The listing builds one solid part. Answer for the finished solid, in the listing's coordinates (mm). Face numbers are marked on the shaded views. A direction names the side the tool comes from. Give positions to 0.01 mm unless a question says otherwise; leave off trailing zeros. Order: outer loops, then holes, each group sorted by start corner. A loop starts at its lowest first (then second) coordinate and runs counter-clockwise, first axis right, second up. Notation, with made-up numbers: (2.5, 1.5) - (58.5, 1.5) arc R34 ccw to (58.5, 38.5) - close; hole circle Ø9 at (80, 64.5). An arc over 180 degrees is marked (long way). Write each question's results on one line, items separated by ' | '. Start each with the question number.
1. Section A-A (z = 13) is taken. Give the vertices of the cut face in (x, y).
2. Which of the six approach directions +Z, -Z, +X, -X, +Y, -Y give full straight-line access (tool end or side, diameter ignored) to the marked faces 1 and 2?
3. Determine the mould class of the marked faces 3, 4, 5 and 6 for opening direction Y: released by +Y, released by -Y, zero draft, split by the parting line, or undercut.
4. Section C-C (x = -5.5) is taken. Give the vertices of the cut face in (y, z), and give its area (3 significant figures).
5. Section D-D (x = -0.25) is taken. Give the vertices of the cut face in (y, z), and give its area (3 significant figures).
6. A flat-ended cylindrical pin translates along its axis: pin 1 (2 mm diameter, centred on y = -0.5, z = 9.5, fed in from -X). Find the tip coordinate at first contact, or state that the pin passes through.
7. Section B-B (y = 0) is taken. Give the vertices of the cut face in (x, z).
8. Find the intervals of material crossed by L1, parallel to Y at x = 6.6, z = 13; L2, parallel to Z at x = 2.75, y = 0.5, in increasing order.
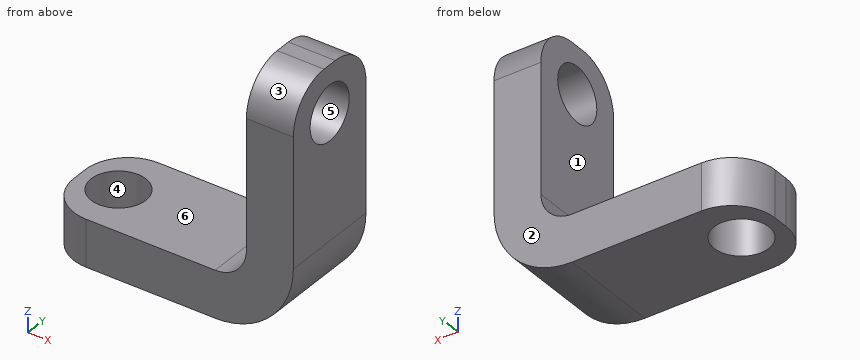
from build123d import *

# Parameters (mm, degrees)
ESQUISSE1_W             = 13
ESQUISSE1_H             = 6.5
ESQUISSE1_R             = 1.75
BOSS_EXTRU_1_DEPTH      = 3
ESQUISSE1_3_W           = 3
ESQUISSE1_3_H           = 6.5
BOSS_EXTRU_2_DEPTH      = 16
ENL_V_MAT_EXTRU_1_REACH = 18
ESQUISSE2_R             = 1.75
CONG_1_R                = 2.75
CONG_2_R                = 2
CONG_3_R                = 5


with BuildPart() as part:
    # Esquisse1 → Boss.-Extru.1 (new body)
    with BuildSketch(Plane.XY):
        with Locations((-1.5, 0)):
            Rectangle(ESQUISSE1_W, ESQUISSE1_H)
        with Locations((-5.5, 0)):
            Circle(ESQUISSE1_R, mode=Mode.SUBTRACT)
    extrude(amount=BOSS_EXTRU_1_DEPTH)

    # Esquisse1_3 → Boss.-Extru.2 (add)
    with BuildSketch(Plane.XY):
        with Locations((6.5, 0)):
            Rectangle(ESQUISSE1_3_W, ESQUISSE1_3_H)
    extrude(amount=BOSS_EXTRU_2_DEPTH)

    # Esquisse2 → Enl_v. mat.-Extru.1 (cut, up to next)
    with BuildSketch(Plane(origin=(8, 0, 0), x_dir=(0, 0, -1), z_dir=(1, 0, 0)), mode=Mode.PRIVATE) as enl_v_mat_extru_1_sk1:
        with Locations((-13, 0)):
            Circle(ESQUISSE2_R)
    enl_v_mat_extru_1_tool1 = extrude(enl_v_mat_extru_1_sk1.sketch, amount=-ENL_V_MAT_EXTRU_1_REACH, mode=Mode.PRIVATE) & part.part
    add(enl_v_mat_extru_1_tool1.solids().sort_by_distance((8, 0, 13))[0], mode=Mode.SUBTRACT)

    # Cong_1
    cong_1_edges = [part.edges().sort_by_distance(p)[0] for p in [
        (-8, 3.25, 1.5),
        (-8, -3.25, 1.5),
        (6.5, 3.25, 16),
        (6.5, -3.25, 16),
    ]]
    fillet(cong_1_edges, radius=CONG_1_R)

    # Cong_2
    cong_2_edges = [part.edges().sort_by_distance(p)[0] for p in [
        (5, 0, 3),
    ]]
    fillet(cong_2_edges, radius=CONG_2_R)

    # Cong_3
    cong_3_edges = [part.edges().sort_by_distance(p)[0] for p in [
        (8, 0, 0),
    ]]
    fillet(cong_3_edges, radius=CONG_3_R)


solid = part.part
Reported:
1) outline: (5, -3.25) - (8, -3.25) - (8, -1.75) - (5, -1.75) - close; (5, 1.75) - (8, 1.75) - (8, 3.25) - (5, 3.25) - close
2) face 1: +Z, -X, +Y, -Y | face 2: +Z, -Z, +X, -X, +Y
3) face 3: released by -Y | face 4: undercut | face 5: undercut | face 6: zero draft
4) outline: (-3.24, 0) - (-1.75, 0) - (-1.75, 3) - (-3.24, 3) - close; (1.75, 0) - (3.24, 0) - (3.24, 3) - (1.75, 3) - close | area: 8.93 mm²
5) outline: (-3.25, 0) - (3.25, 0) - (3.25, 3) - (-3.25, 3) - close | area: 19.5 mm²
6) pin 1: x = 5
7) outline: (-8, 0) - (-7.25, 0) - (-7.25, 3) - (-8, 3) - close; (-3.75, 0) - (3, 0) arc R5 ccw to (8, 5) - (8, 11.25) - (5, 11.25) - (5, 5) arc R2 cw to (3, 3) - (-3.75, 3) - close; (5, 14.75) - (8, 14.75) - (8, 16) - (5, 16) - close
8) L1: -3.25 to -1.75, 1.75 to 3.25 | L2: 0 to 3
